```python
from build123d import *

# Parameters (mm, degrees)
SKETCH_1_W      = 54.3
SKETCH_1_H      = 57.8
EXTRUDE_1_DEPTH = 30
EXTRUDE_2_DEPTH = 3
FILLET_1_R      = 2.5


with BuildPart() as part:
    # Эскиз1 → Бобышка-Вытянуть1 (new body)
    with BuildSketch(Plane.XY.offset(-7)):
        with BuildLine():
            Line((-26.25, -31), (26.25, -31))
            ThreePointArc((26.25, -31), (28.371320344, -30.121320344), (29.25, -28))
            Line((29.25, -28), (29.25, 28))
            ThreePointArc((29.25, 28), (28.371320344, 30.121320344), (26.25, 31))
            Line((26.25, 31), (-26.25, 31))
            ThreePointArc((-26.25, 31), (-28.371320344, 30.121320344), (-29.25, 28))
            Line((-29.25, 28), (-29.25, -28))
            ThreePointArc((-29.25, -28), (-28.371320344, -30.121320344), (-26.25, -31))
        make_face()
        Rectangle(SKETCH_1_W, SKETCH_1_H, mode=Mode.SUBTRACT)
    extrude(amount=EXTRUDE_1_DEPTH)

    # Эскиз2 → Бобышка-Вытянуть2 (add)
    with BuildSketch(Plane.XY.offset(23)):
        with BuildLine():
            Line((-26.25, -31), (26.25, -31))
            ThreePointArc((26.25, -31), (28.371320344, -30.121320344), (29.25, -28))
            Line((29.25, -28), (29.25, 28))
            ThreePointArc((29.25, 28), (28.371320344, 30.121320344), (26.25, 31))
            Line((26.25, 31), (-26.25, 31))
            ThreePointArc((-26.25, 31), (-28.371320344, 30.121320344), (-29.25, 28))
            Line((-29.25, 28), (-29.25, -28))
            ThreePointArc((-29.25, -28), (-28.371320344, -30.121320344), (-26.25, -31))
        make_face()
    extrude(amount=EXTRUDE_2_DEPTH)

    # Скругление1
    fillet_1_edges = [part.edges().sort_by_distance(p)[0] for p in [
        (0, 28.9, 23),
        (-27.15, 0, 23),
        (0, -28.9, 23),
        (27.15, 0, 23),
    ]]
    fillet(fillet_1_edges, radius=FILLET_1_R)


solid = part.part
```
Input: part model. Units: mm. Frame: model coordinates. A direction names the side the tool comes from. Round coordinates to 2 decimals unless told otherwise and drop trailing zeros. Loops run counter-clockwise (first coordinate to the right, second up) from the corner with the lowest first, then second, coordinate; pieces in that order, holes last. Notation, with made-up numbers: (87.5, -1) - (116.5, -1) arc R21 cw to (116.5, 24) - close; hole circle Ø2 at (76, 6.25). An arc over 180 degrees is marked (long way). One line per item, written item: value. Start each with the question number.
(1) Draft query along X for faces 1 (the cylindrical face through (28.35, -30.14, 9.27)), 2 (the flat face through (-27.15, 0, 7)), 3 (the cylindrical face through (-28.39, -30.1, 9.27)). Return one class per face: +X half, -X half, draft (parallel to the pull), parting line (faces both ways), or undercut.
(2) Ray query, line 1 (Y direction, x = 23, z = 0); line 2 (X direction, y = 3.5, z = -3); line 3 (Z direction, x = 8, y = 26.5). Return the intervals inside material, ascending. Write a range as [from, to].
(3) Access query for faces 4 (the cylindrical face through (28.39, 30.1, 9.27)), 5 (the flat face through (0, -28.9, 7)). Directions: +Z, -Z, +X, -X, +Y, -Y. A direction counts if a zero-diameter tool reaches every point of the face in a straight line with its end or side. Return the directions, or none.
(4) Section B-B, the plane y = -9. Return loops of the section in (x, z), plus the area to 3 significant figures.
(5) Section A-A, the plane z = 14.5. Return loops of the section in (x, y), plus the area to 3 significant figures.
(6) Contact query for a flat-ended pin moving along its axis: P1, Ø3, axis at x = -5, y = 9.5, coming from the -Z side. Output: stop coordinate, or through.
Results below:
1. face 1: +X half
1. face 2: undercut
1. face 3: -X half
2. line 1: [-31, -28.9], [28.9, 31]
2. line 2: [-29.25, -27.15], [27.15, 29.25]
2. line 3: [23, 26]
3. face 4: +Z, -Z, +X, +Y
3. face 5: -Z
4. outline: (-29.25, -7) - (-27.15, -7) - (-27.15, 20.5) arc R2.5 cw to (-24.65, 23) - (24.65, 23) arc R2.5 cw to (27.15, 20.5) - (27.15, -7) - (29.25, -7) - (29.25, 26) - (-29.25, 26) - close
4. area: 304 mm^2
5. outline: (-29.25, -28) arc R3 ccw to (-26.25, -31) - (26.25, -31) arc R3 ccw to (29.25, -28) - (29.25, 28) arc R3 ccw to (26.25, 31) - (-26.25, 31) arc R3 ccw to (-29.25, 28) - close; hole (-27.15, -28.9) - (27.15, -28.9) - (27.15, 28.9) - (-27.15, 28.9) - close
5. area: 481 mm^2
6. P1: z = 23
